from build123d import *

# Parameters (mm, degrees)
SKETCH_1_W               = 100
SKETCH_1_H               = 130
EXTRUDE_1_DEPTH          = 3
SKETCH_2_R               = 2.1
CUT_EXTRUDE_1_DEPTH      = 83.060952956
SKETCH_5_W               = 100
SKETCH_5_H               = 130
EXTRUDE_2_DEPTH          = 3
CUT_EXTRUDE_4_DEPTH      = 164.505351594
CUT_EXTRUDE_4_DEPTH_BACK = 164.505351594
SKETCH_6_R               = 2.1
CUT_EXTRUDE_5_DEPTH      = 164.505351594
CUT_EXTRUDE_5_DEPTH_BACK = 164.505351594
SKETCH_7_R               = 2.55
CUT_EXTRUDE_6_DEPTH      = 164.505351594
CUT_EXTRUDE_6_DEPTH_BACK = 164.505351594
SKETCH_8_W               = 200
SKETCH_8_H               = 20


with BuildPart() as part:
    # 草图1 → 凸台-拉伸1 (new body)
    with BuildSketch(Plane.XY):
        Rectangle(SKETCH_1_W, SKETCH_1_H)
    extrude(amount=EXTRUDE_1_DEPTH)

    # 草图2 → 切除-拉伸1 (cut, through all)
    with BuildSketch(Plane.XY.offset(3)):
        with Locations((-40, 55)):
            Circle(SKETCH_2_R)
        with Locations((-20, 55)):
            Circle(SKETCH_2_R)
        with Locations((0, 55)):
            Circle(SKETCH_2_R)
        with Locations((20, 55)):
            Circle(SKETCH_2_R)
        with Locations((40, 55)):
            Circle(SKETCH_2_R)
        with Locations((-40, 0)):
            Circle(SKETCH_2_R)
        with Locations((-40, -55)):
            Circle(SKETCH_2_R)
        with Locations((-40, -110)):
            Circle(SKETCH_2_R)
        with Locations((-40, -165)):
            Circle(SKETCH_2_R)
        with Locations((-40, -220)):
            Circle(SKETCH_2_R)
        with Locations((-40, -275)):
            Circle(SKETCH_2_R)
        with Locations((-40, -330)):
            Circle(SKETCH_2_R)
        with Locations((-40, -385)):
            Circle(SKETCH_2_R)
        with Locations((40, -385)):
            Circle(SKETCH_2_R)
        with Locations((40, -330)):
            Circle(SKETCH_2_R)
        with Locations((40, -275)):
            Circle(SKETCH_2_R)
        with Locations((40, -220)):
            Circle(SKETCH_2_R)
        with Locations((40, -165)):
            Circle(SKETCH_2_R)
        with Locations((40, -110)):
            Circle(SKETCH_2_R)
        with Locations(Location((40, -55, 0), (0, 0, 180))):
            Circle(SKETCH_2_R)
        with Locations(Location((40, 0, 0), (0, 0, 180))):
            Circle(SKETCH_2_R)
        with Locations(Location((20, -55, 0), (0, 0, 180))):
            Circle(SKETCH_2_R)
        with Locations(Location((0, -55, 0), (0, 0, 180))):
            Circle(SKETCH_2_R)
        with Locations(Location((-20, -55, 0), (0, 0, 180))):
            Circle(SKETCH_2_R)
    extrude(amount=-CUT_EXTRUDE_1_DEPTH, mode=Mode.SUBTRACT)

    # 草图5 → 凸台-拉伸2 (add)
    with BuildSketch(Plane.XY.offset(3)):
        with Locations((100, 0)):
            Rectangle(SKETCH_5_W, SKETCH_5_H)
    extrude(amount=-EXTRUDE_2_DEPTH)

    # 草图6 → 切除-拉伸4 (cut, two sides: drawn at the far end of the back side and taken through both)
    with BuildSketch(Plane.XY.offset(3).offset(-CUT_EXTRUDE_4_DEPTH_BACK)):
        with Locations((55, 55)):
            Circle(SKETCH_6_R)
        with Locations((70, 55)):
            Circle(SKETCH_6_R)
        with Locations((85, 55)):
            Circle(SKETCH_6_R)
        with Locations((100, 55)):
            Circle(SKETCH_6_R)
        with Locations((115, 55)):
            Circle(SKETCH_6_R)
        with Locations((130, 55)):
            Circle(SKETCH_6_R)
        with Locations((145, 55)):
            Circle(SKETCH_6_R)
        with Locations((145, -55)):
            Circle(SKETCH_6_R)
        with Locations((130, -55)):
            Circle(SKETCH_6_R)
        with Locations((115, -55)):
            Circle(SKETCH_6_R)
        with Locations((100, -55)):
            Circle(SKETCH_6_R)
        with Locations((85, -55)):
            Circle(SKETCH_6_R)
        with Locations((70, -55)):
            Circle(SKETCH_6_R)
        with Locations((55, -55)):
            Circle(SKETCH_6_R)
    extrude(amount=CUT_EXTRUDE_4_DEPTH + CUT_EXTRUDE_4_DEPTH_BACK, mode=Mode.SUBTRACT)

    # 草图7 → 切除-拉伸5 (cut, two sides: drawn at the far end of the back side and taken through both)
    with BuildSketch(Plane(origin=(0, 0, 0), x_dir=(-1, 0, 0), z_dir=(0, 0, -1)).offset(-CUT_EXTRUDE_5_DEPTH_BACK)):
        with Locations((-140, -30)):
            Circle(SKETCH_7_R)
        with Locations((-120, -30)):
            Circle(SKETCH_7_R)
        with Locations((-100, -30)):
            Circle(SKETCH_7_R)
        with Locations((-80, -30)):
            Circle(SKETCH_7_R)
        with Locations((-60, -30)):
            Circle(SKETCH_7_R)
        with Locations((-40, -30)):
            Circle(SKETCH_7_R)
        with Locations((-20, -30)):
            Circle(SKETCH_7_R)
        with Locations((0, -30)):
            Circle(SKETCH_7_R)
        with Locations((20, -30)):
            Circle(SKETCH_7_R)
        with Locations((40, -30)):
            Circle(SKETCH_7_R)
    extrude(amount=CUT_EXTRUDE_5_DEPTH + CUT_EXTRUDE_5_DEPTH_BACK, mode=Mode.SUBTRACT)

    # 草图8 → 切除-拉伸6 (cut, two sides: drawn at the far end of the back side and taken through both)
    with BuildSketch(Plane(origin=(0, 0, 0), x_dir=(-1, 0, 0), z_dir=(0, 0, -1)).offset(-CUT_EXTRUDE_6_DEPTH_BACK)):
        with Locations((-50, -55)):
            Rectangle(SKETCH_8_W, SKETCH_8_H)
    extrude(amount=CUT_EXTRUDE_6_DEPTH + CUT_EXTRUDE_6_DEPTH_BACK, mode=Mode.SUBTRACT)


solid = part.part
Model file for the job. Use its own axes, mm. Give positions to 0.01 mm unless a question says otherwise; leave off trailing zeros. Loops run counter-clockwise (first coordinate to the right, second up) from the corner with the lowest first, then second, coordinate; pieces in that order, holes last. Notation, with made-up numbers: (-10, 88) - (36, 88) arc R35 cw to (36, 122) - close; hole circle Ø9 at (78, 1). An arc over 180 degrees is marked (long way). Use one line per item in the form item = value.
(1) Cut at D-D (x = 0). Give the cut face in (y, z), then the cut area to 3 significant figures.
Determined:
outline = (-45, 0) - (-32.55, 0) - (-32.55, 3) - (-45, 3) - close; (-27.45, 0) - (52.9, 0) - (52.9, 3) - (-27.45, 3) - close; (57.1, 0) - (65, 0) - (65, 3) - (57.1, 3) - close
area = 302 mm^2
(2) Cut at C-C (z = 0.55). Count the separate pieces of the cut face and the enclosed holes in it, then the cut area to 3 significant figures.
Determined:
separate_pieces = 1
enclosed_holes = 24
area = 21,600 mm^2
(3) Pull direction Y, two halves, no side cores. Call faces 1 (the face through (49, 11, 0)), 2 (the face through (137.57, -29.23, 1.52)): pulls with the +Y half, pulls with the -Y half, needs draft (parallel to the pull), parting line crosses it, or undercut.
Determined:
face_1 = needs draft
face_2 = undercut
(4) Cut at A-A (x = -40). Give the cut face in (y, z).
Determined:
outline = (-45, 0) - (-32.55, 0) - (-32.55, 3) - (-45, 3) - close; (-27.45, 0) - (-2.1, 0) - (-2.1, 3) - (-27.45, 3) - close; (2.1, 0) - (52.9, 0) - (52.9, 3) - (2.1, 3) - close; (57.1, 0) - (65, 0) - (65, 3) - (57.1, 3) - close
(5) Cut at B-B (x = 55). Give the cut face in (y, z), then the cut area to 3 significant figures.
Determined:
outline = (-45, 0) - (52.9, 0) - (52.9, 3) - (-45, 3) - close; (57.1, 0) - (65, 0) - (65, 3) - (57.1, 3) - close
area = 317 mm^2
(6) Drill centre lines: L1, parallel to Y at x = 0, z = 2.05; L2, parallel to Y at x = -40, z = 1.2; L3, parallel to Y at x = 145, z = 1.5. Where is each one in solid material? Low to high.
Determined:
L1 = -45 to -32.55, -27.45 to 52.9, 57.1 to 65
L2 = -45 to -32.55, -27.45 to -2.1, 2.1 to 52.9, 57.1 to 65
L3 = -45 to 52.9, 57.1 to 65
